Read the model definition and answer for the solid it produces. Units are mm, in the model's axes. Face numbers are marked on the shaded views. A direction names the side the tool comes from. Round coordinates to 2 decimals unless told otherwise and drop trailing zeros. Order: outer loops, then holes, each group sorted by start corner. A loop starts at its lowest first (then second) coordinate and runs counter-clockwise, first axis right, second up. Notation, with made-up numbers: (-11.75, -24) - (47.25, -24) arc R24 ccw to (47.25, 15) - close; hole circle Ø6 at (54, 78.5). An arc over 180 degrees is marked (long way). Answer as a JSON object with one key per item and string values. Group by question number.
Q1. Given pin 1 Ø4 at (x, y) = (-5, -9) entering from +Z; pin 2 Ø6 at (y, z) = (-0.5, 8) entering from +X, each flat-ended and moving along its own axis, determine where each tip first touches the part or whether it passes through.
Q2. A tool of negligible diameter and unlimited length cuts with its end or side. For the marked faces 1 and 2, from which of +Z, -Z, +X, -X, +Y, -Y can it reach the whole face along a straight path? Write none if from no direction.
Q3. A cutting plane is placed at D-D on y = 9.5. Determine the outline of the cut face in (x, z) (3 decimals).
Q4. A cutting plane is placed at C-C on z = 8. Determine the outline of the cut face in (x, y) (3 decimals), and give its area (3 significant figures).
Q5. Consider line 1 (Z direction, x = 8, y = 13.5); line 2 (Z direction, x = 3.75, y = -0.5); line 3 (Y direction, x = -3, z = 1). Determine where each line is inside the solid, lowest interval first.
```python
from build123d import *

# Parameters (mm, degrees)
F0_R     = 5.9055
F1_DEPTH = 6.223
F2_R     = 3.175
F3_DEPTH = 19.05
F5_DEPTH = 31.75


with BuildPart() as f1:
    # F0 (on Top) → F1 (new body)
    with BuildSketch(Plane.XY):
        Circle(F0_R)
    extrude(amount=F1_DEPTH)

    # F2 (on face) → F3 (join)
    with BuildSketch(Plane.XY.offset(6.223)):
        Circle(F2_R)
    extrude(amount=F3_DEPTH)

    # F4 (on face) → F5 (join)
    with BuildSketch(Plane(origin=(0, 0, 0), x_dir=(1, 0, 0), z_dir=(0, 0, -1))):
        Polygon((9.525, -16.637), (-9.525, 16.637), (-9.525, -16.637), align=None)
        Polygon((9.525, 16.637), (-9.525, 16.637), (9.525, -16.637), align=None)
    extrude(amount=F5_DEPTH)


solid = f1.part
```
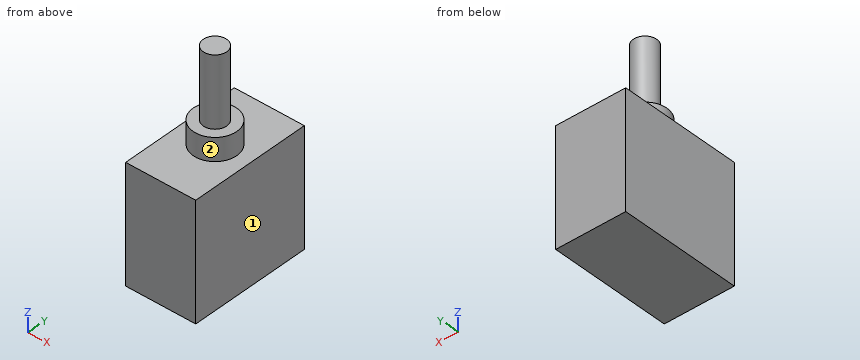
Result set:
{
 "1": {"pin 1": "stops at z = 0", "pin 2": "stops at x = 5.91"},
 "2": {"face 1": "+Z, -Z, +X, +Y, -Y", "face 2": "+Z"},
 "3": {"outline": "(-9.525, -31.75) - (9.525, -31.75) - (9.525, 0) - (-9.525, 0) - close"},
 "4": {"outline": "circle Ø6.35 at (0, 0)", "area": "31.7 mm²"},
 "5": {"line 1": "z = -31.75 to 0", "line 2": "z = -31.75 to 6.22", "line 3": "y = -5.09 to 5.09"}
}
